Can you work these out from the model? Positions are in its coordinate system, mm. A direction names the side the tool comes from. Coordinates: 2 decimals unless noted, no trailing zeros. Loops run counter-clockwise (first coordinate to the right, second up) from the corner with the lowest first, then second, coordinate; pieces in that order, holes last. Notation, with made-up numbers: (89, 72) -> (110, 72) arc R34 cw to (110, 104) -> close; hole circle Ø7 at (13.25, 54.5). An arc over 180 degrees is marked (long way). Put each result on its own line as item: value. Start each with the question number.
Item 1: If we section it at A-A on z = 35: Please give me the cut outline in (x, y), plus the area to 4 significant figures.
Item 2: Please list where these lines run through material, in increasing order: L1, parallel to X at y = 1.3, z = 10; L2, parallel to X at y = 3.9, z = 35; L3, parallel to Y at x = 7.5, z = 36. Write a range as from..to.
Item 3: For faces 1 (the cylindrical face through (6.67, 1.232, 61.617)), 2 (the flat face through (8, 2.5, 135)), which set-ups out of +Z, -Z, +X, -X, +Y, -Y let a thin tool reach every point of the face, with its end or its side?
Item 4: If we section it at B-B on y = 4.75: Please give me the cut outline in (x, z).
Item 5: We'd pull the mould along X, two halves only. Please class faces 3 (the flat face through (6, 0, 71)), 4 (the flat face through (0, 4, 71)), 5 (the flat face through (8, 2.5, 85)), 6 (the flat face through (12, 4, 71)): pulls with the +X half, pulls with the -X half, needs draft (parallel to the pull), parting line crosses it, or undercut.
Item 6: If we section it at D-D on z = 109.5: Please give me the cut outline in (x, y), plus the area to 3 significant figures.
Item 7: If we section it at C-C on x = 6: State how many separate pieces and enclosed holes the cut face has, plus the area to 3 significant figures.
Item 8: Will this pin go through, and if not, where does the flat tip stop? P1, Ø1.8, axis at x = 4.5, z = 110.5, coming from the +Y side.
Autodesk Inventor part; units mm, degrees
ref_plane "YZ Plane" through (0, 0, 0) normal (1, 0, 0) x (0, 1, 0)
ref_plane "XZ Plane" through (0, 0, 0) normal (0, 1, 0) x (-1, 0, 0)
ref_plane "XY Plane" through (0, 0, 0) normal (0, 0, 1) x (1, 0, 0)
sketch "スケッチ1" plane through (0, 0, 0) normal (0, 0, 1) x (1, 0, 0)
  line L0 (0, 0) -> (12, 0)
  line L1 (12, 0) -> (12, 7.5)
  line L2 (12, 7.5) -> (0, 7.5)
  line L3 (0, 7.5) -> (0, 0)
  dimension "d0" = 12
  dimension "d1" = 7.5
extrude "押し出し1" add sketch "スケッチ1" along normal blind 145
sketch "スケッチ2" plane through (0, 7.5, 0) normal (0, 1, 0) x (1, 0, 0)
  line L0 (12, -145) -> (0, -145)
  line L1 (6, -145) -> (6, 0)
  line L2 (12, 0) -> (0, 0)
  point P0 (6, -10)
  point P1 (6, -135)
  point P2 (6, -110)
  point P3 (6, -85)
  point P4 (6, -60)
  point P5 (6, -35)
  dimension "d4" = 10
  dimension "d5" = 10
  dimension "d6" = 25
  dimension "d7" = 25
  dimension "d8" = 25
  dimension "d9" = 25
  dimension "d10" = 25
hole "穴1" at (6, 7.5, 10) at (6, 7.5, 135) at (6, 7.5, 110) at (6, 7.5, 85) at (6, 7.5, 60) at (6, 7.5, 35) direction (0, -1, 0) diameter 3.5 end through all
sketch "スケッチ3" plane through (0, 7.5, 0) normal (0, 1, 0) x (1, 0, 0)
  line L0 (12, -145) -> (0, -145)
  line L1 (6, -145) -> (6, 0)
  line L2 (12, 0) -> (0, 0)
  point P0 (6, -10)
  point P1 (6, -135)
  point P2 (6, -110)
  point P3 (6, -85)
  point P4 (6, -60)
  point P5 (6, -35)
  dimension "d18" = 10
  dimension "d19" = 10
  dimension "d20" = 25
  dimension "d21" = 25
  dimension "d22" = 25
  dimension "d23" = 25
  dimension "d24" = 25
hole "穴2" at (6, 7.5, 10) at (6, 7.5, 135) at (6, 7.5, 110) at (6, 7.5, 60) at (6, 7.5, 35) at (6, 7.5, 85) direction (0, -1, 0) diameter 6 depth 5
properties part number "slider" material "アルミニウム 6061-AHC"
Solutions:
1. outline: (0, 0) -> (4.25, 0) -> (4.25, 2.5) -> (3, 2.5) -> (3, 7.5) -> (0, 7.5) -> close; (7.75, 0) -> (12, 0) -> (12, 7.5) -> (9, 7.5) -> (9, 2.5) -> (7.75, 2.5) -> close
1. area: 51.25 mm^2
2. L1: 0..4.25, 7.75..12
2. L2: 0..3, 9..12
2. L3: 0..2.5
3. face 1: +Y, -Y
3. face 2: +Y
4. outline: (0, 0) -> (12, 0) -> (12, 145) -> (0, 145) -> close; hole circle Ø6 at (6, 10); hole circle Ø6 at (6, 35); hole circle Ø6 at (6, 60); hole circle Ø6 at (6, 85); hole circle Ø6 at (6, 110); hole circle Ø6 at (6, 135)
5. face 3: needs draft
5. face 4: pulls with the -X half
5. face 5: undercut
5. face 6: pulls with the +X half
6. outline: (0, 0) -> (4.32, 0) -> (4.32, 2.5) -> (3.04, 2.5) -> (3.04, 7.5) -> (0, 7.5) -> close; (7.68, 0) -> (12, 0) -> (12, 7.5) -> (8.96, 7.5) -> (8.96, 2.5) -> (7.68, 2.5) -> close
6. area: 52.0 mm^2
7. separate pieces: 7
7. enclosed holes: 0
7. area: 855 mm^2
8. P1: y = 2.5
